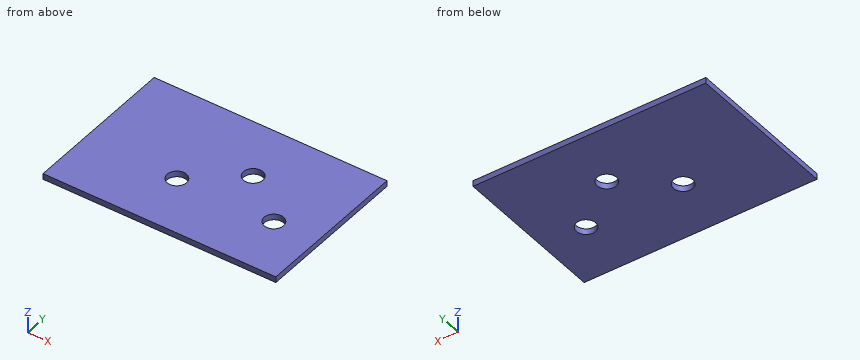
Autodesk Inventor part; units mm, degrees
ref_plane "YZ Plane" through (0, 0, 0) normal (1, 0, 0) x (0, 1, 0)
ref_plane "XZ Plane" through (0, 0, 0) normal (0, 1, 0) x (-1, 0, 0)
ref_plane "XY Plane" through (0, 0, 0) normal (0, 0, 1) x (1, 0, 0)
sketch "Sketch1" plane through (0, 0, 0) normal (0, 0, 1) x (1, 0, 0)
  line L0 (-19.5625, -111.2599) -> (-19.5625, 1344.9999)
  line L1 (40.4374, -111.2599) -> (40.4374, 1344.9999)
  line L2 (14.1874, 432.5) -> (19.1874, 432.5)
  line L3 (19.1874, 427.5) -> (14.1874, 427.5)
  line L4 (26.6874, 422.5) -> (31.6874, 422.5)
  line L5 (31.6874, 417.5) -> (26.6874, 417.5)
  line L6 (1.6874, 422.5) -> (6.6874, 422.5)
  line L7 (6.6874, 417.5) -> (1.6874, 417.5)
  line L8 (4.1874, 417.5) -> (4.1874, 422.5) construction
  line L9 (16.6874, 427.5) -> (16.6874, 432.5) construction
  line L10 (29.1874, 417.5) -> (29.1874, 422.5) construction
  circle A0 centre (4.1874, 420) radius 2.5
  circle A1 centre (16.6874, 430) radius 2.5
  circle A2 centre (29.1874, 420) radius 2.5
  line L11 (40.4374, 405) -> (-19.5625, 405)
  line L12 (-19.5625, 405) -> (-19.5625, 445)
  line L13 (-19.5625, 445) -> (40.4374, 445)
  line L14 (40.4374, 445) -> (40.4374, 405)
  point P0 (0, 0)
  dimension "d0" = 15
  dimension "d1" = 15
extrude "Plate1" add sketch "Sketch1" along normal blind 1.5
equation "\"BendRadius\" = Thickness"
equation "\"BendReliefWidth\" = Thickness"
equation "\"BendReliefDepth\" = 0.5 * Thickness"
equation "\"CornerReliefSize\" = 4 * Thickness"
equation "\"MinimumRemnant\" = 2 * Thickness"
equation "\"TransitionRadius\" = BendRadius"
equation "\"JacobiRadiusSize\" = BendRadius"
equation "\"GapSize\" = Thickness"
equation "\"d2\" = BendRadius"
properties part number "gabarito-porta-cabos" material "Wood (Oak)"
Verification items for the finished model (mm, model axes). Coordinates: 2 decimals unless noted, no trailing zeros. Order: outer loops, then holes, each group sorted by start corner. A loop starts at its lowest first (then second) coordinate and runs counter-clockwise, first axis right, second up. Notation, with made-up numbers: M 70,-17.75 L 84,-17.75 A8 cw 84,-5.75 Z; hole C -19.5,40.5 d4. An arc over 180 degrees is marked long. One line per item, written item: value. Start each with the question number.
Item 1: Sectioned sample at C-C on y = 420. Record the cut outline in (x, z), then the cut area to 3 significant figures.
Item 2: Sectioned sample at A-A on y = 430. Record the cut outline in (x, z), then the cut area to 3 significant figures.
Item 3: Sectioned sample at B-B on z = 0.8. Record the cut outline in (x, y), then the cut area to 3 significant figures.
Item 4: Thickness scan on probe 1 along X at (y, z) = (420, 0.45); probe 2 along X at (y, z) = (420.5, 0.65); probe 3 along X at (y, z) = (430, 1.05). Record the ranges inside material, lowest first.
Calculated:
1. outline: M -19.56,0 L 1.69,0 L 1.69,1.5 L -19.56,1.5 Z; M 6.69,0 L 26.69,0 L 26.69,1.5 L 6.69,1.5 Z; M 31.69,0 L 40.44,0 L 40.44,1.5 L 31.69,1.5 Z
1. area: 75.0 mm^2
2. outline: M -19.56,0 L 14.19,0 L 14.19,1.5 L -19.56,1.5 Z; M 19.19,0 L 40.44,0 L 40.44,1.5 L 19.19,1.5 Z
2. area: 82.5 mm^2
3. outline: M -19.56,405 L 40.44,405 L 40.44,445 L -19.56,445 Z; hole C 4.19,420 d5; hole C 16.69,430 d5; hole C 29.19,420 d5
3. area: 2,340 mm^2
4. probe 1: -19.56 to 1.69, 6.69 to 26.69, 31.69 to 40.44
4. probe 2: -19.56 to 1.74, 6.64 to 26.74, 31.64 to 40.44
4. probe 3: -19.56 to 14.19, 19.19 to 40.44
